```python
from build123d import *

# Parameters (mm, degrees)
SKETCH1_W           = 46
SKETCH1_H           = 40
BOSS_EXTRUDE1_DEPTH = 40
SKETCH2_W           = 46
SKETCH2_H           = 3.7
BOSS_EXTRUDE2_DEPTH = 16
SKETCH5_W           = 40
SKETCH5_H           = 34
CUT_EXTRUDE3_DEPTH  = 37
FILLET1_R           = 1
FILLET2_R           = 1
CUT_EXTRUDE6_DEPTH  = 3.5
SKETCH9_W           = 46
SKETCH9_H           = 1
BOSS_EXTRUDE3_DEPTH = 2
CUT_EXTRUDE7_REACH  = 65.551
SKETCH12_R          = 2.1
CUT_EXTRUDE8_REACH  = 55.429
SKETCH13_R          = 2.1
FILLET3_R           = 2


with BuildPart() as part:
    # Sketch1 → Boss-Extrude1 (new body)
    with BuildSketch(Plane(origin=(0, 0, 0), x_dir=(1, 0, 0), z_dir=(0, 1, 0))):
        Rectangle(SKETCH1_W, SKETCH1_H)
    extrude(amount=BOSS_EXTRUDE1_DEPTH)

    # Sketch2 → Boss-Extrude2 (add)
    with BuildSketch(Plane.XZ):
        with Locations((0, 21.85)):
            Rectangle(SKETCH2_W, SKETCH2_H)
        with Locations((0, -21.85)):
            Rectangle(SKETCH2_W, SKETCH2_H)
    extrude(amount=-BOSS_EXTRUDE2_DEPTH)

    # Sketch5 → Cut-Extrude3 (cut)
    with BuildSketch(Plane.XZ):
        Rectangle(SKETCH5_W, SKETCH5_H)
    extrude(amount=-CUT_EXTRUDE3_DEPTH, mode=Mode.SUBTRACT)

    # Fillet1
    fillet1_edges = [part.edges().sort_by_distance(p)[0] for p in [
        (23, 40, 0),
        (0, 40, -20),
        (-23, 16, 21.85),
        (23, 16, 21.85),
        (0, 16, 20),
        (-23, 16, -21.85),
        (0, 16, -20),
        (23, 16, -21.85),
        (-23, 40, 0),
        (0, 40, 20),
        (-23, 28, -20),
        (23, 28, -20),
        (23, 28, 20),
        (-23, 28, 20),
    ]]
    fillet(fillet1_edges, radius=FILLET1_R)

    # Fillet2
    fillet2_edges = [part.edges().sort_by_distance(p)[0] for p in [
        (-20, 37, 0),
        (-20, 18.5, -17),
        (0, 37, 17),
        (-20, 18.5, 17),
        (20, 37, 0),
        (20, 18.5, 17),
        (0, 37, -17),
        (20, 18.5, -17),
    ]]
    fillet(fillet2_edges, radius=FILLET2_R)

    # Sketch3 → Cut-Extrude6 (cut)
    with BuildSketch(Plane(origin=(0, 0, -23.7), x_dir=(-1, 0, 0), z_dir=(0, 0, -1))):
        Polygon((2.078460969, 11.6), (-2.078460969, 11.6), (-4.156921938, 8), (-2.078460969, 4.4), (2.078460969, 4.4), (4.156921938, 8), align=None)
    cut_extrude6 = extrude(amount=-CUT_EXTRUDE6_DEPTH, mode=Mode.SUBTRACT)

    # Mirror2: Cut-Extrude6 across plane
    add(cut_extrude6.mirror(Plane.XY), mode=Mode.SUBTRACT)

    # Sketch9 → Boss-Extrude3 (add)
    with BuildSketch(Plane.XZ):
        with Locations((0, 20.7)):
            Rectangle(SKETCH9_W, SKETCH9_H)
        with Locations((0, -20.7)):
            Rectangle(SKETCH9_W, SKETCH9_H)
    extrude(amount=BOSS_EXTRUDE3_DEPTH)

    # Sketch12 → Cut-Extrude7 (cut, up to next)
    with BuildSketch(Plane.XY.offset(20), mode=Mode.PRIVATE) as cut_extrude7_sk1:
        with Locations((0, 24)):
            Circle(SKETCH12_R)
    cut_extrude7_tool1 = extrude(cut_extrude7_sk1.sketch, amount=-CUT_EXTRUDE7_REACH, mode=Mode.PRIVATE) & part.part
    add(cut_extrude7_tool1.solids().sort_by_distance((0, 24, 20))[0], mode=Mode.SUBTRACT)

    # Sketch13 → Cut-Extrude8 (cut, up to next)
    with BuildSketch(Plane(origin=(0, 40, 0), x_dir=(1, 0, 0), z_dir=(0, 1, 0)), mode=Mode.PRIVATE) as cut_extrude8_sk1:
        with Locations(Location((0, 10, 0), (0, 0, 270))):
            Circle(SKETCH13_R)
    cut_extrude8_tool1 = extrude(cut_extrude8_sk1.sketch, amount=-CUT_EXTRUDE8_REACH, mode=Mode.PRIVATE) & part.part
    add(cut_extrude8_tool1.solids().sort_by_distance((0, 40, -10))[0], mode=Mode.SUBTRACT)

    # Fillet3
    fillet3_edges = [part.edges().sort_by_distance(p)[0] for p in [
        (0, 0, 21.2),
        (0, 0, -21.2),
    ]]
    fillet(fillet3_edges, radius=FILLET3_R - 0.0001)  # a hair under: the kernel refuses the full size


solid = part.part
```
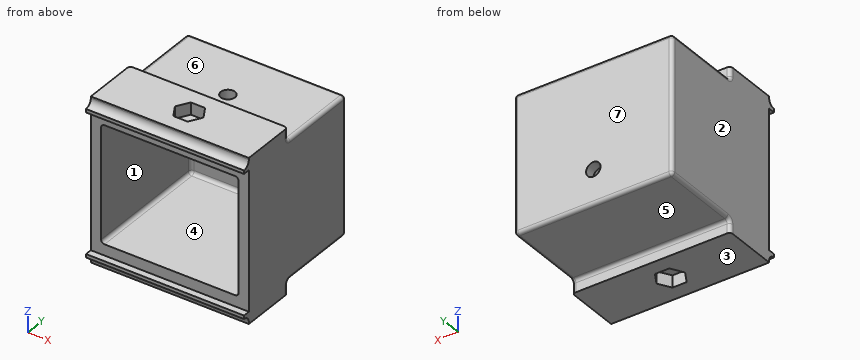
Design review of the part built by this model. Coordinates are the model's own, in mm. Face numbers are marked on the shaded views. A direction names the side the tool comes from. Coordinates: 2 decimals unless noted, no trailing zeros. Order: outer loops, then holes, each group sorted by start corner. A loop starts at its lowest first (then second) coordinate and runs counter-clockwise, first axis right, second up. Notation, with made-up numbers: M -38,-9.75 L 13,-9.75 A13 ccw 13,4.25 Z; hole C 70,-29 d9. An arc over 180 degrees is marked long. Answer as a JSON object with one key per item and string values. Group by question number.
1) Add section D-D, the plane y = 24. Write out the cut boundary in (x, z), then the cut area to 3 significant figures.
2) Mouldability with a two-part tool opening along X and no side actions: class the marked faces 1, 2, 3 and 4 as pulls with the +X half, pulls with the -X half, needs draft (parallel to the pull), parting line crosses it, or undercut.
3) Add section A-A, the plane z = -10. Write out the cut boundary in (x, y).
4) Add section B-B, the plane y = 30.5. Write out the cut boundary in (x, z), then the cut area to 3 significant figures.
5) For pin 1 (6 mm diameter, centred on x = -17, y = 28.5, fed in from -Z); pin 2 (4 mm diameter, centred on x = 2.5, z = 13, fed in from -Y); pin 3 (1.4 mm diameter, centred on x = 0.5, z = -23, fed in from +Y), all flat-tipped, find the tip position at first contact; note any pin that passes through.
6) Tool access review of the marked faces 5, 6 and 7: name each direction out of +Z, -Z, +X, -X, +Y, -Y from which nothing blocks a thin tool from reaching the whole face with its end or side.
7) Wall thickness on L1, parallel to Z at x = 18.5, y = 31.5; L2, parallel to X at y = 16.5, z = -7; L3, parallel to Z at x = -4, y = 5.5: over which ranges is each line inside the solid? List them lowest first.
Computed values:
{
 "1": {"outline": "M -23,-19 A1 ccw -22,-20 L 22,-20 A1 ccw 23,-19 L 23,19 A1 ccw 22,20 L 2.1,20 L 2.1,17 L 19,17 A1 cw 20,16 L 20,-16 A1 cw 19,-17 L -19,-17 A1 cw -20,-16 L -20,16 A1 cw -19,17 L -2.1,17 L -2.1,20 L -22,20 A1 ccw -23,19 Z", "area": "467 mm^2"},
 "2": {"face 1": "undercut", "face 2": "pulls with the -X half", "face 3": "needs draft", "face 4": "undercut"},
 "3": {"outline": "M -23,0 L -20,0 L -20,36 A1 cw -19,37 L -2.1,37 L -2.1,40 L -22,40 A1 ccw -23,39 Z; M 2.1,37 L 19,37 A1 cw 20,36 L 20,0 L 23,0 L 23,39 A1 ccw 22,40 L 2.1,40 Z"},
 "4": {"outline": "M -23,-19 A1 ccw -22,-20 L 22,-20 A1 ccw 23,-19 L 23,19 A1 ccw 22,20 L -22,20 A1 ccw -23,19 Z; hole M -20,-16 A1 ccw -19,-17 L 19,-17 A1 ccw 20,-16 L 20,16 A1 ccw 19,17 L -19,17 A1 ccw -20,16 Z", "area": "480 mm^2"},
 "5": {"pin 1": "stops at z = -20", "pin 2": "stops at y = 37", "pin 3": "stops at y = 16"},
 "6": {"face 5": "-Z, +X, -X, +Y", "face 6": "+Z, +X, -X, +Y", "face 7": "+Z, -Z, +X, -X, +Y"},
 "7": {"L1": "z = -20 to -17, 17 to 20", "L2": "x = -23 to -20, 20 to 23", "L3": "z = -23.7 to -17, 17 to 23.7"}
}
